```python
from build123d import *

# Parameters (mm, degrees)
SKETCH1_W           = 100
SKETCH1_H           = 100
BOSS_EXTRUDE1_DEPTH = 53.5
SKETCH2_R           = 2.5
SKETCH2_W           = 12.6
SKETCH2_H           = 3.072407599
BOSS_EXTRUDE2_DEPTH = 4
CUT_EXTRUDE1_DEPTH  = 47.5
FILLET1_R           = 3.25
FILLET2_R           = 3
SKETCH4_R           = 1.625
CUT_EXTRUDE2_DEPTH  = 14
FILLET3_R           = 3
BOSS_EXTRUDE3_START = 6.5
SKETCH8_R           = 1.625
BOSS_EXTRUDE3_DEPTH = 6.5
SKETCH10_W          = 159.412029064
SKETCH10_H          = 131.965012122
CUT_EXTRUDE3_DEPTH  = 205.5
SKETCH11_R          = 1.625
CUT_EXTRUDE4_DEPTH  = 2.8
FILLET4_R           = 1.5
FILLET5_R           = 0.5
BOSS_EXTRUDE4_DEPTH = 5
FILLET6_R           = 0.5
CUT_EXTRUDE5_DEPTH  = 130
CUT_EXTRUDE6_DEPTH  = 130


with BuildPart() as part:
    # Sketch1 → Boss-Extrude1 (new body)
    with BuildSketch(Plane(origin=(0, 0, 0), x_dir=(1, 0, 0), z_dir=(0, 1, 0))):
        Rectangle(SKETCH1_W, SKETCH1_H)
    extrude(amount=BOSS_EXTRUDE1_DEPTH)

    # Sketch2 → Boss-Extrude2 (add)
    # profile 1 of 8: a face of its own
    with BuildSketch(Plane.XZ):
        with BuildLine():
            Line((33.15, -50), (20.55, -50))
            Line((20.55, -50), (20.55, -56.973787721))
            ThreePointArc((20.55, -56.973787721), (26.85, -63.273787721), (33.15, -56.973787721))
            Line((33.15, -56.973787721), (33.15, -50))
        make_face()
        with Locations(Location((26.85, -56.973787721, 0), (0, 0, 270))):
            Circle(SKETCH2_R, mode=Mode.SUBTRACT)
    # profile 2 of 8: a face of its own
    with BuildSketch(Plane.XZ):
        with BuildLine():
            Line((-20.55, -56.973787721), (-20.55, -50))
            Line((-20.55, -50), (-33.15, -50))
            Line((-33.15, -50), (-33.15, -56.973787721))
            ThreePointArc((-33.15, -56.973787721), (-26.85, -63.273787721), (-20.55, -56.973787721))
        make_face()
        with Locations(Location((-26.85, -56.973787721, 0), (0, 0, 270))):
            Circle(SKETCH2_R, mode=Mode.SUBTRACT)
    # profile 3 of 8: a face of its own
    with BuildSketch(Plane.XZ):
        with Locations((-26.85, 48.4637962)):
            Rectangle(SKETCH2_W, SKETCH2_H)
    # profile 4 of 8: a face of its own
    with BuildSketch(Plane.XZ):
        with BuildLine():
            Line((-33.15, 50), (-20.55, 50))
            Line((-20.55, 50), (-20.55, 56.973787721))
            ThreePointArc((-20.55, 56.973787721), (-26.85, 63.273787721), (-33.15, 56.973787721))
            Line((-33.15, 56.973787721), (-33.15, 50))
        make_face()
        with Locations(Location((-26.85, 56.973787721, 0), (0, 0, 270))):
            Circle(SKETCH2_R, mode=Mode.SUBTRACT)
    # profile 5 of 8: a face of its own
    with BuildSketch(Plane.XZ):
        with BuildLine():
            Line((20.55, 56.973787721), (20.55, 50))
            Line((20.55, 50), (33.15, 50))
            Line((33.15, 50), (33.15, 56.973787721))
            ThreePointArc((33.15, 56.973787721), (26.85, 63.273787721), (20.55, 56.973787721))
        make_face()
        with Locations(Location((26.85, 56.973787721, 0), (0, 0, 270))):
            Circle(SKETCH2_R, mode=Mode.SUBTRACT)
    # profile 6 of 8: a face of its own
    with BuildSketch(Plane.XZ):
        with Locations((26.85, 48.4637962)):
            Rectangle(SKETCH2_W, SKETCH2_H)
    # profile 7 of 8: a face of its own
    with BuildSketch(Plane.XZ):
        with Locations((26.85, -48.4637962)):
            Rectangle(SKETCH2_W, SKETCH2_H)
    # profile 8 of 8: a face of its own
    with BuildSketch(Plane.XZ):
        with Locations((-26.85, -48.4637962)):
            Rectangle(SKETCH2_W, SKETCH2_H)
    extrude(amount=-BOSS_EXTRUDE2_DEPTH)

    # Sketch3 → Cut-Extrude1 (cut)
    with BuildSketch(Plane(origin=(0, 53.5, 0), x_dir=(1, 0, 0), z_dir=(0, 1, 0))):
        Polygon((35.565, 48), (-35.565, 48), (-48, 35.565), (-48, -35.565), (-35.565, -48), (35.565, -48), (48, -35.565), (48, 35.565), align=None)
    extrude(amount=-CUT_EXTRUDE1_DEPTH, mode=Mode.SUBTRACT)

    # Fillet1
    fillet1_edges = [part.edges().sort_by_distance(p)[0] for p in [
        (50, 26.75, 50),
        (-50, 26.75, 50),
        (-50, 26.75, -50),
        (50, 26.75, -50),
    ]]
    fillet(fillet1_edges, radius=FILLET1_R)

    # Fillet2
    fillet2_edges = [part.edges().sort_by_distance(p)[0] for p in [
        (-26.85, 4, 50),
        (26.85, 4, 50),
        (26.85, 4, -50),
        (-26.85, 4, -50),
    ]]
    fillet(fillet2_edges, radius=FILLET2_R)

    # Sketch4 → Cut-Extrude2 (cut)
    with BuildSketch(Plane(origin=(0, 53.5, 0), x_dir=(1, 0, 0), z_dir=(0, 1, 0))):
        with Locations(Location((-46.75, 46.75, 0), (0, 0, 270))):
            Circle(SKETCH4_R)
        with Locations(Location((46.75, 46.75, 0), (0, 0, 270))):
            Circle(SKETCH4_R)
        with Locations(Location((46.75, -46.75, 0), (0, 0, 270))):
            Circle(SKETCH4_R)
        with Locations(Location((-46.75, -46.75, 0), (0, 0, 270))):
            Circle(SKETCH4_R)
    extrude(amount=-CUT_EXTRUDE2_DEPTH, mode=Mode.SUBTRACT)

    # Fillet3
    fillet3_edges = [part.edges().sort_by_distance(p)[0] for p in [
        (50, 0, 0),
        (39.95, 0, -50),
        (-39.95, 0, 50),
        (-50, 0, 0),
        (49.048097039, 0, -49.048097039),
        (-49.048097039, 0, -49.048097039),
        (-49.048097039, 0, 49.048097039),
        (49.048097039, 0, 49.048097039),
        (0, 0, 50),
        (39.95, 0, 50),
        (0, 0, -50),
        (-39.95, 0, -50),
    ]]
    fillet(fillet3_edges, radius=FILLET3_R)

    # Sketch8 → Boss-Extrude3 (add)
    # profile 1 of 2: a face of its own
    with BuildSketch(Plane(origin=(0, 53.5, 0), x_dir=(1, 0, 0), z_dir=(0, 1, 0)).offset(BOSS_EXTRUDE3_START)):
        with BuildLine():
            ThreePointArc((-50, -46.75), (-49.048097039, -49.048097039), (-46.75, -50))
            Line((-46.75, -50), (46.75, -50))
            ThreePointArc((46.75, -50), (49.048097039, -49.048097039), (50, -46.75))
            Line((50, -46.75), (50, 46.75))
            ThreePointArc((50, 46.75), (49.048097039, 49.048097039), (46.75, 50))
            Line((46.75, 50), (-46.75, 50))
            ThreePointArc((-46.75, 50), (-49.048097039, 49.048097039), (-50, 46.75))
            Line((-50, 46.75), (-50, -46.75))
        make_face()
        with Locations(Location((-46.75, 46.75, 0), (0, 0, 270))):
            Circle(SKETCH8_R, mode=Mode.SUBTRACT)
        with Locations(Location((46.75, 46.75, 0), (0, 0, 270))):
            Circle(SKETCH8_R, mode=Mode.SUBTRACT)
        with Locations(Location((-46.75, -46.75, 0), (0, 0, 270))):
            Circle(SKETCH8_R, mode=Mode.SUBTRACT)
        with Locations(Location((46.75, -46.75, 0), (0, 0, 270))):
            Circle(SKETCH8_R, mode=Mode.SUBTRACT)
        Polygon((-35.565, 48), (35.565, 48), (48, 35.565), (48, -35.565), (35.565, -48), (-35.565, -48), (-48, -35.565), (-48, 35.565), align=None, mode=Mode.SUBTRACT)
    # profile 2 of 2: a face of its own
    with BuildSketch(Plane(origin=(0, 53.5, 0), x_dir=(1, 0, 0), z_dir=(0, 1, 0)).offset(BOSS_EXTRUDE3_START)):
        Polygon((35.565, 48), (48, 35.565), (48, -35.565), (35.565, -48), (-35.565, -48), (-48, -35.565), (-48, 35.565), (-35.565, 48), align=None)
    extrude(amount=-BOSS_EXTRUDE3_DEPTH)

    # Sketch10 → Cut-Extrude3 (cut)
    with BuildSketch(Plane.XZ.offset(-53.5)):
        Rectangle(SKETCH10_W, SKETCH10_H)
    extrude(amount=CUT_EXTRUDE3_DEPTH, mode=Mode.SUBTRACT)

    # Sketch11 → Cut-Extrude4 (cut)
    # profile 1 of 4: a face of its own
    with BuildSketch(Plane(origin=(0, 60, 0), x_dir=(1, 0, 0), z_dir=(0, 1, 0))):
        with BuildLine():
            Line((-46.75, -41.75), (-50, -41.75))
            Line((-50, -41.75), (-50, -46.75))
            ThreePointArc((-50, -46.75), (-49.048097039, -49.048097039), (-46.75, -50))
            Line((-46.75, -50), (-41.75, -50))
            Line((-41.75, -50), (-41.75, -46.75))
            ThreePointArc((-41.75, -46.75), (-43.214466094, -43.214466094), (-46.75, -41.75))
        make_face()
        with Locations(Location((-46.75, -46.75, 0), (0, 0, 270))):
            Circle(SKETCH11_R, mode=Mode.SUBTRACT)
    # profile 2 of 4: a face of its own
    with BuildSketch(Plane(origin=(0, 60, 0), x_dir=(1, 0, 0), z_dir=(0, 1, 0))):
        with BuildLine():
            Line((-50, 41.75), (-46.75, 41.75))
            ThreePointArc((-46.75, 41.75), (-43.214466094, 43.214466094), (-41.75, 46.75))
            Line((-41.75, 46.75), (-41.75, 50))
            Line((-41.75, 50), (-46.75, 50))
            ThreePointArc((-46.75, 50), (-49.048097039, 49.048097039), (-50, 46.75))
            Line((-50, 46.75), (-50, 41.75))
        make_face()
        with Locations(Location((-46.75, 46.75, 0), (0, 0, 270))):
            Circle(SKETCH11_R, mode=Mode.SUBTRACT)
    # profile 3 of 4: a face of its own
    with BuildSketch(Plane(origin=(0, 60, 0), x_dir=(1, 0, 0), z_dir=(0, 1, 0))):
        with BuildLine():
            Line((46.75, 50), (41.75, 50))
            Line((41.75, 50), (41.75, 46.75))
            ThreePointArc((41.75, 46.75), (43.214466094, 43.214466094), (46.75, 41.75))
            Line((46.75, 41.75), (50, 41.75))
            Line((50, 41.75), (50, 46.75))
            ThreePointArc((50, 46.75), (49.048097039, 49.048097039), (46.75, 50))
        make_face()
        with Locations(Location((46.75, 46.75, 0), (0, 0, 270))):
            Circle(SKETCH11_R, mode=Mode.SUBTRACT)
    # profile 4 of 4: a face of its own
    with BuildSketch(Plane(origin=(0, 60, 0), x_dir=(1, 0, 0), z_dir=(0, 1, 0))):
        with BuildLine():
            Line((41.75, -46.75), (41.75, -50))
            Line((41.75, -50), (46.75, -50))
            ThreePointArc((46.75, -50), (49.048097039, -49.048097039), (50, -46.75))
            Line((50, -46.75), (50, -41.75))
            Line((50, -41.75), (46.75, -41.75))
            ThreePointArc((46.75, -41.75), (43.214466094, -43.214466094), (41.75, -46.75))
        make_face()
        with Locations(Location((46.75, -46.75, 0), (0, 0, 270))):
            Circle(SKETCH11_R, mode=Mode.SUBTRACT)
    extrude(amount=-CUT_EXTRUDE4_DEPTH, mode=Mode.SUBTRACT)

    # Fillet4
    fillet4_edges = [part.edges().sort_by_distance(p)[0] for p in [
        (0, 60, 50),
        (50, 60, 0),
        (0, 60, -50),
        (-50, 60, 0),
        (48.375, 60, 41.75),
        (41.75, 60, 48.375),
        (43.214466094, 60, 43.214466094),
        (43.214466094, 60, -43.214466094),
        (48.375, 60, -41.75),
        (41.75, 60, -48.375),
        (-48.375, 60, -41.75),
        (-41.75, 60, -48.375),
        (-43.214466094, 60, -43.214466094),
        (-43.214466094, 60, 43.214466094),
        (-48.375, 60, 41.75),
        (-41.75, 60, 48.375),
    ]]
    fillet(fillet4_edges, radius=FILLET4_R)

    # Fillet5
    fillet5_edges = [part.edges().sort_by_distance(p)[0] for p in [
        (50, 57.2, 44.25),
        (49.048097039, 57.2, 49.048097039),
        (44.25, 57.2, 50),
        (44.25, 57.2, -50),
        (49.048097039, 57.2, -49.048097039),
        (50, 57.2, -44.25),
        (-50, 57.2, -44.25),
        (-49.048097039, 57.2, -49.048097039),
        (-44.25, 57.2, -50),
        (-44.25, 57.2, 50),
        (-49.048097039, 57.2, 49.048097039),
        (-50, 57.2, 44.25),
    ]]
    fillet(fillet5_edges, radius=FILLET5_R)

    # Sketch12 → Boss-Extrude4 (add)
    with BuildSketch(Plane.XZ.offset(-53.5)):
        Polygon((-45.3, -34.446623382), (-34.446623382, -45.3), (34.446623382, -45.3), (45.3, -34.446623382), (45.3, 34.446623382), (34.446623382, 45.3), (-34.446623382, 45.3), (-45.3, 34.446623382), align=None)
        Polygon((-33.411089476, -42.8), (33.411089476, -42.8), (42.8, -33.411089476), (42.8, 33.411089476), (33.411089476, 42.8), (-33.411089476, 42.8), (-42.8, 33.411089476), (-42.8, -33.411089476), align=None, mode=Mode.SUBTRACT)
    extrude(amount=BOSS_EXTRUDE4_DEPTH)

    # Fillet6
    fillet6_edges = [part.edges().sort_by_distance(p)[0] for p in [
        (0, 53.5, -42.8),
        (38.105544738, 53.5, -38.105544738),
        (42.8, 53.5, 0),
        (38.105544738, 53.5, 38.105544738),
        (0, 53.5, 42.8),
        (-38.105544738, 53.5, 38.105544738),
        (-42.8, 53.5, 0),
        (-38.105544738, 53.5, -38.105544738),
    ]]
    fillet(fillet6_edges, radius=FILLET6_R)

    # Sketch13 → Cut-Extrude5 (cut)
    with BuildSketch(Plane.ZY.offset(45.3)):
        Polygon((-34.446623382, 48.5), (-26.446623382, 50.5), (26.446623382, 50.5), (34.446623382, 48.5), align=None)
    extrude(amount=-CUT_EXTRUDE5_DEPTH, mode=Mode.SUBTRACT)

    # Sketch14 → Cut-Extrude6 (cut)
    with BuildSketch(Plane.XY.offset(45.3)):
        Polygon((-34.446623382, 48.5), (-26.700656689, 50.5), (28.522356043, 50.5), (36.268322735, 48.5), align=None)
    extrude(amount=-CUT_EXTRUDE6_DEPTH, mode=Mode.SUBTRACT)


solid = part.part
```
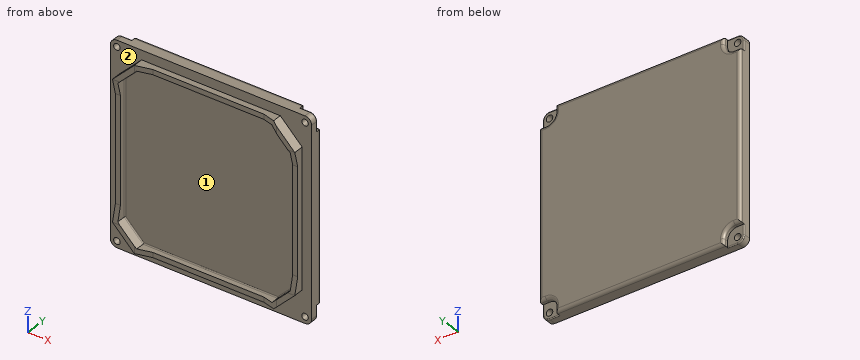
The model under review builds one solid part; all positions refer to its coordinate system, in mm. Face numbers are marked on the shaded views. Round coordinates to 2 decimals unless told otherwise and drop trailing zeros. Loops run counter-clockwise (first coordinate to the right, second up) from the corner with the lowest first, then second, coordinate; pieces in that order, holes last. Notation, with made-up numbers: (13, 6) - (22, 6) arc R29 cw to (22, 42) - close; hole circle Ø8 at (7.25, 13). An arc over 180 degrees is marked (long way). Use a Markdown table: item, result. Add a question column.
Q1. Add section B-B (x = 20.5). State the section outline as (y, z) points.
Q2. Add section A-A (z = -6). State the section outline as (x, y) points.
Q3. For probe 1 along X at (y, z) = (55.15, 46.75) (3 decimals); probe 2 along Y at (x, z) = (-26, -27); probe 3 along Y at (x, z) = (-14, -43), list the stretches that pass through material, from the lowest coordinate up.
Q4. Insertion check: pin 1 Ø0.5 at (x, y) = (-48.5, 58) entering from +Z; pin 2 Ø1.5 at (y, z) = (52, 7.5) entering from -X; pin 3 Ø6 at (x, z) = (-44, -47.5) entering from +Y; pin 4 Ø3 at (x, z) = (-46.75, -46.75) entering from +Y. Each pin has a flat end and moves straight along its axis. Give the tip position at first contact, or say it passes through.
Q5. The part is to be moulded in two halves that separate along Z. For the marked faces 1 and 2, say which applies: pulls with the +Z half, pulls with the -Z half, needs draft (parallel to the pull), parting line crosses it, or undercut.
Worked answers:
| question | item | result |
|---|---|---|
| 1 | outline | (50.5, -45.3) - (53.5, -45.3) - (53.5, -50) - (58.5, -50) arc R1.5 ccw to (60, -48.5) - (60, 48.5) arc R1.5 ccw to (58.5, 50) - (53.5, 50) - (53.5, 45.3) - (50.5, 45.3) - (50.5, 42.8) - (53, 42.8) arc R0.5 cw to (53.5, 42.3) - (53.5, -42.3) arc R0.5 cw to (53, -42.8) - (50.5, -42.8) - close |
| 2 | outline | (-50, 53.5) - (-45.3, 53.5) - (-45.3, 50.5) - (-42.8, 50.5) - (-42.8, 53) arc R0.5 cw to (-42.3, 53.5) - (42.3, 53.5) arc R0.5 cw to (42.8, 53) - (42.8, 50.5) - (45.3, 50.5) - (45.3, 53.5) - (50, 53.5) - (50, 58.5) arc R1.5 ccw to (48.5, 60) - (-48.5, 60) arc R1.5 ccw to (-50, 58.5) - close |
| 3 | probe 1 | -50 to -48.375, -45.125 to 45.125, 48.375 to 50 |
| 3 | probe 2 | 53.5 to 60 |
| 3 | probe 3 | 50.5 to 60 |
| 4 | pin 1 | z = 41.75 |
| 4 | pin 2 | x = -45.3 |
| 4 | pin 3 | y = 59.8 |
| 4 | pin 4 | through |
| 5 | face 1 | undercut |
| 5 | face 2 | needs draft |
